Job drawing, mm, ordinate dimensions from the low corner. One solid piece. A direction names the side the tool comes from. Give positions to 0.01 mm unless a question says otherwise; leave off trailing zeros. Loops run counter-clockwise (first coordinate to the right, second up) from the corner with the lowest first, then second, coordinate; pieces in that order, holes last. Notation, with made-up numbers: (18.25, -35) - (76.25, -35) arc R26 ccw to (76.25, -8) - close; hole circle Ø6 at (9, -18.5). An arc over 180 degrees is marked (long way). Answer as CSV lines item,"result". Start each with the question number.
Item 1: Saw through at C-C on y = 5.5. Give the cut face in (x, z), plus the area to 3 significant figures.
Item 2: Pull direction Z, two halves, no side cores. Call the marked faces 4, 5, 6 and 7: pulls with the +Z half, pulls with the -Z half, needs draft (parallel to the pull), parting line crosses it, or undercut.
Item 3: Tool access for the marked faces 1, 2 and 3: list every direction of +Z, -Z, +X, -X, +Y, -Y with a clear straight run to the whole face (end or side of a thin tool).
Item 4: Saw through at D-D on z = 24. Give the cut face in (x, y), plus the area to 3 significant figures.
Item 5: Saw through at B-B on x = 40. Give the cut face in (y, z), plus the area to 3 significant figures.
Item 6: Saw through at A-A on z = 12.5. Give the cut face in (x, y), plus the area to 3 significant figures.
Item 7: Drill centre lines: L1, parallel to X at y = 13.75, z = 20; L2, parallel to Z at x = 43, y = 2.5; L3, parallel to Z at x = 37.5, y = 2. Where is each one in solid material? Low to high. Write a range as from..to.
Item 8: Pin check, flat tips, straight feed: pin 1 (1 mm diameter, centred on x = 31.5, z = 19.5, fed in from -Y); pin 2 (1 mm diameter, centred on x = 8.5, y = 2, fed in from +Z); pin 3 (3 mm diameter, centred on y = 15, z = 33, fed in from -X). Stop position of each tip, or through.
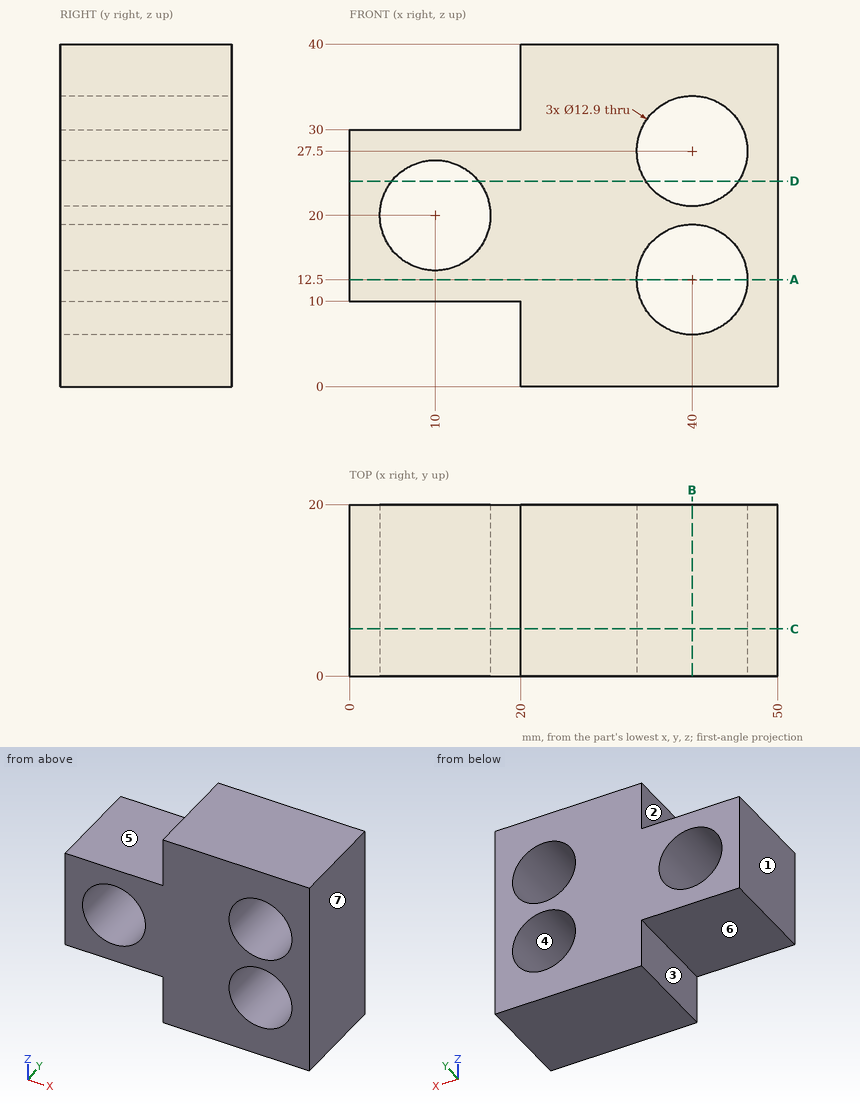
Responses:
1,outline,"(0, 10) - (20, 10) - (20, 0) - (50, 0) - (50, 40) - (20, 40) - (20, 30) - (0, 30) - close; hole circle Ø12.9 at (10, 20); hole circle Ø12.9 at (40, 12.5); hole circle Ø12.9 at (40, 27.5)"
1,area,"1,210 mm2"
2,face 4,"undercut"
2,face 5,"pulls with the +Z half"
2,face 6,"pulls with the -Z half"
2,face 7,"needs draft"
3,face 1,"+Z, -Z, -X, +Y, -Y"
3,face 2,"+Z, -X, +Y, -Y"
3,face 3,"-Z, -X, +Y, -Y"
4,outline,"(0, 0) - (4.94, 0) - (4.94, 20) - (0, 20) - close; (15.06, 0) - (34.58, 0) - (34.58, 20) - (15.06, 20) - close; (45.42, 0) - (50, 0) - (50, 20) - (45.42, 20) - close"
4,area,"581 mm2"
5,outline,"(0, 0) - (20, 0) - (20, 6.05) - (0, 6.05) - close; (0, 18.95) - (20, 18.95) - (20, 21.05) - (0, 21.05) - close; (0, 33.95) - (20, 33.95) - (20, 40) - (0, 40) - close"
5,area,"284 mm2"
6,outline,"(0, 0) - (33.55, 0) - (33.55, 20) - (0, 20) - close; (46.45, 0) - (50, 0) - (50, 20) - (46.45, 20) - close"
6,area,"742 mm2"
7,L1,"0..3.55, 16.45..50"
7,L2,"0..6.79, 18.21..21.79, 33.21..40"
7,L3,"0..6.55, 18.45..21.55, 33.45..40"
8,pin 1,"y = 0"
8,pin 2,"z = 30"
8,pin 3,"x = 20"
